Model file for the job. Use its own axes, mm. A direction names the side the tool comes from. Round coordinates to 2 decimals unless told otherwise and drop trailing zeros. Loops run counter-clockwise (first coordinate to the right, second up) from the corner with the lowest first, then second, coordinate; pieces in that order, holes last. Notation, with made-up numbers: M 75.5,72.25 L 102.5,72.25 A9 ccw 102.5,78.25 Z; hole C 88,-5 d10. An arc over 180 degrees is marked long. Use a Markdown table: item, result. Add a question column.
Item 1: Saw through at C-C on y = 25. Write the cut outline in (x, z), then the cut area to 3 significant figures.
Item 2: Tool access for faces 1 (the flat face through (43.58, -29.68, 121.6)), 2 (the flat face through (0, -8, 223)), 3 (the flat face through (54.37, 12.59, 123.93)), 4 (the flat face through (53.755, -20.782, 110.278)): list every direction of +Z, -Z, +X, -X, +Y, -Y with a clear straight run to the whole face (end or side of a thin tool).
Item 3: Wall check: L1, parallel to Z at x = 19.5, y = -0.5; L2, parallel to X at y = -8, z = 214; L3, parallel to Y at x = -0.5, z = 50. Give the ranges that are in metal, low to high. Write a range as from..to.
Item 4: Saw through at B-B on z = 195.5. Write the cut outline in (x, y).
Item 5: Saw through at A-A on x = 45.5. Write the cut outline in (y, z).
Item 6: Saw through at D-D on x = 57.5. Write the cut outline in (y, z).
Item 7: Pin check, flat tips, straight feed: P1, Ø1, axis at x = 38.5, y = 0, coming from the +Z side; P2, Ø12, axis at y = 18.5, z = 69.5, coming from the -X side; P3, Ø8, axis at y = 8, z = 49.5, coming from the +X side; P4, Ø24, axis at x = -0.5, y = 1.5, coming from the +Z side. Stop position of each tip, or through.
```python
from build123d import *

# Parameters (mm, degrees)
F0_R     = 39.9204473095
F1_DEPTH = 203.2
F2_W     = 19.8161117733
F2_H     = 16.0770136863
F3_DEPTH = 39.37
F5_DEPTH = 71.882
F7_DEPTH = 15.494


with BuildPart() as f1:
    # F0 (on Top) → F1 (new body)
    with BuildSketch(Plane.XY):
        Circle(F0_R)
    extrude(amount=F1_DEPTH)

    # F2 (on face) → F3 (join)
    with BuildSketch(Plane.XY.offset(203.2)):
        with Locations((-9.9080558866, -8.0385068431)):
            Rectangle(F2_W, F2_H)
    extrude(amount=F3_DEPTH)

    # F4 (on face) → F5 (join)
    with BuildSketch(Plane.YZ):
        Polygon((-11.0862118476, 102.8951700695), (11.0862118476, 112.177238249), (14.1339168521, 136.0201545224), (-4.9908018387, 150.5810026161), (-27.1632255339, 141.2989344366), (-30.2109305384, 117.4560181633), align=None)
    extrude(amount=F5_DEPTH)

    # F6 (on face) → F7 (cut)
    with BuildSketch(Plane(origin=(0, -44.4976190456, 5.6878787267), x_dir=(1, 0, 0), z_dir=(0, -0.9919292372, 0.1267926987))):
        with BuildLine():
            ThreePointArc((41.2940425882, 136.7144455761), (46.1384221296, 116.821871488), (62.9989352422, 128.4367591143))
            ThreePointArc((62.9989352422, 128.4367591143), (62.182928441, 132.8663777994), (59.8420390413, 136.7144455761))
            Line((59.8420390413, 136.7144455761), (41.2940425882, 136.7144455761))
        make_face()
    extrude(amount=-F7_DEPTH, mode=Mode.SUBTRACT)


solid = f1.part
```
Entries:
| question | item | result |
|---|---|---|
| 1 | outline | M -31.12,0 L 31.12,0 L 31.12,203.2 L -31.12,203.2 Z |
| 1 | area | 12,600 mm2 |
| 2 | face 1 | +Z, +X, -Y |
| 2 | face 2 | +Z, +X, +Y, -Y |
| 2 | face 3 | -Z, +X, +Y |
| 2 | face 4 | -Z, +X, -Y |
| 3 | L1 | 0..203.2 |
| 3 | L2 | -19.82..0 |
| 3 | L3 | -39.92..39.92 |
| 4 | outline | C 0,0 d79.84 |
| 5 | outline | M -30.21,117.46 L -11.09,102.9 L 11.09,112.18 L 14.13,136.02 L -4.99,150.58 L -27.16,141.3 L -11.79,139.33 L -14.28,119.86 L -29.65,121.83 Z |
| 6 | outline | M -30.21,117.46 L -11.09,102.9 L 11.09,112.18 L 14.13,136.02 L -4.99,150.58 L -27.16,141.3 L -11.79,139.33 L -14.15,120.89 L -29.52,122.85 Z |
| 7 | P1 | z = 203.2 |
| 7 | P2 | x = -37.91 |
| 7 | P3 | x = 39.72 |
| 7 | P4 | z = 242.57 |
